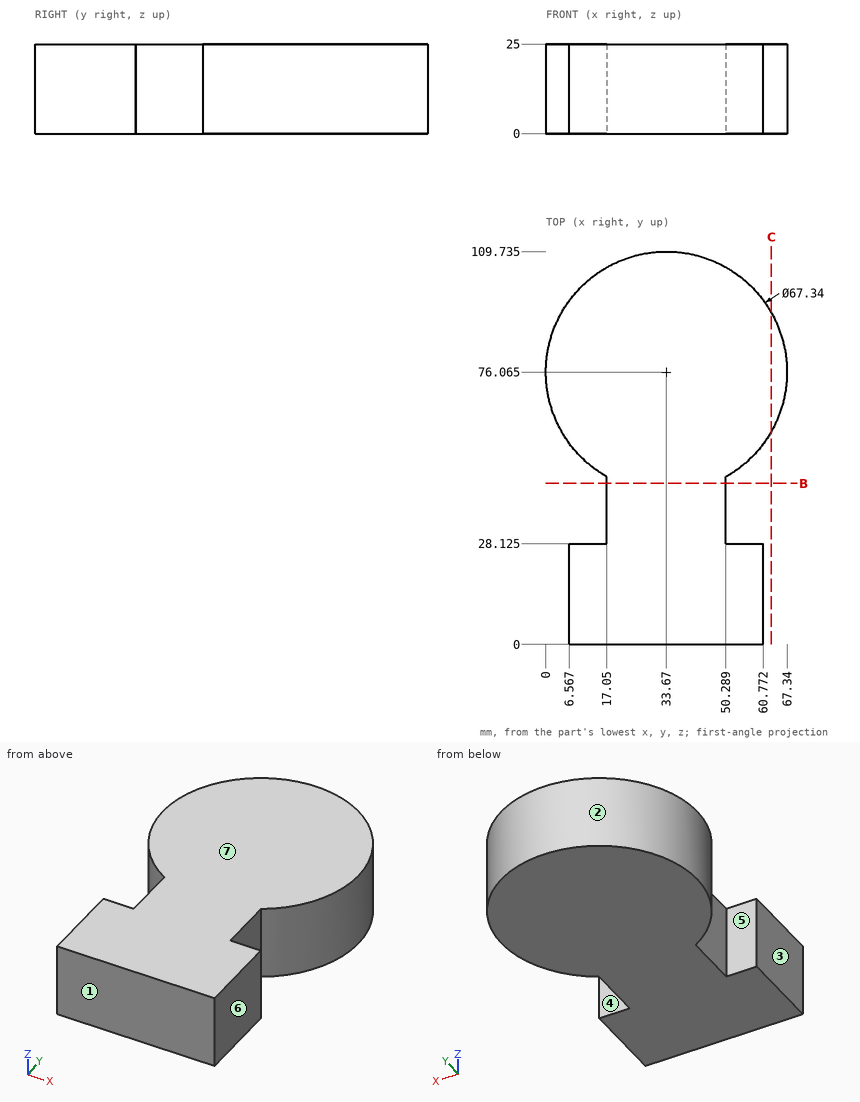
Answer from the drawing. Dimensions are ordinates in mm from the lowest x, y and z of the part. A direction names the side the tool comes from. Give positions to 0.01 mm unless a question says otherwise; leave off trailing zeros. Write each loop counter-clockwise with the first axis right and the second up, starting at its lowest first coordinate (ties: lowest second). Pieces come first, ordered by that corner, then holes. Notation, with made-up numbers: (19.25, 5) - (34.25, 5) arc R7 ccw to (34.25, 14) - close; hole circle Ø8 at (9, 35). An arc over 180 degrees is marked (long way). One line per item, written item: value. Start each with the question number.
1. Given pin 1 (9.5 mm diameter, centred on y = 35, z = 8.5, fed in from +X); pin 2 (7.5 mm diameter, centred on y = 20.5, z = 13.5, fed in from -X); pin 3 (3 mm diameter, centred on y = 98, z = 5.5, fed in from +X); pin 4 (8 mm diameter, centred on x = 51.5, y = 37.5, fed in from -Z), each flat-ended and moving along its own axis, determine where each tip first touches the part or whether it passes through.
2. For the marked faces 4, 5, 6 and 7, determine the directions among +Z, -Z, +X, -X, +Y, -Y from which every point of the face is accessible in a straight line to the end or side of a thin tool.
3. For a pull along Y with two mould halves and no side action, classify the marked faces 1, 2 and 3 as +Y half, -Y half, draft (parallel to the pull), parting line (faces both ways), or undercut.
4. Find section C-C (x = 63). Write down the section's boundary in (y, z).
5. Consider probe 1 along X at (y, z) = (45, 15.5); probe 2 along Y at (x, z) = (33, 17.25); probe 3 along X at (y, z) = (21, 23.5). Determine where each line is inside the solid, lowest interval first.
6. Find section B-B (y = 45). Write down the section's boundary in (x, z).
Geometry results:
1. pin 1: x = 50.29
1. pin 2: x = 6.57
1. pin 3: x = 60.43
1. pin 4: z = 0
2. face 4: +Z, -Z, +X
2. face 5: +Z, -Z, -X
2. face 6: +Z, -Z, +X, -Y
2. face 7: +Z, +X, -X, +Y, -Y
3. face 1: -Y half
3. face 2: undercut
3. face 3: draft
4. outline: (59.53, 0) - (92.6, 0) - (92.6, 25) - (59.53, 25) - close
5. probe 1: 17.05 to 50.29
5. probe 2: 0 to 109.73
5. probe 3: 6.57 to 60.77
6. outline: (17.05, 0) - (50.29, 0) - (50.29, 25) - (17.05, 25) - close
